Read the model definition and answer for the solid it produces. Units are mm, in the model's axes. A direction names the side the tool comes from. Give positions to 0.01 mm unless a question says otherwise; leave off trailing zeros. Loops run counter-clockwise (first coordinate to the right, second up) from the corner with the lowest first, then second, coordinate; pieces in that order, holes last. Notation, with made-up numbers: (7.25, -35.5) - (57.25, -35.5) arc R31 ccw to (57.25, -5.5) - close; hole circle Ø11 at (57.5, 6.25). An arc over 180 degrees is marked (long way). Put each result on its own line as item: value. Start each with the question number.
1. For faces 4 (the cylindrical face through (78.4, 0.18, 46.79)), 5 (the flat face through (76.835, -26, -25)), determine the directions among +Z, -Z, +X, -X, +Y, -Y from which every point of the face is accessible in a straight line to the end or side of a thin tool.
2. For a pull along Z with two mould halves and no side action, classify faces 1 (the flat face through (67.31, -18, 65)), 2 (the flat face through (80.01, 44, 1)), 3 (the cylindrical face through (1.12, -22.025, -99.184)) as released by +Z, released by -Z, zero draft, split by the parting line, or undercut.
3. Given pin 1 Ø6 at (x, z) = (13.5, 31) entering from -Y; pin 2 Ø8 at (x, y) = (-53, 69) entering from -Z; pin 3 Ø2 at (x, z) = (36.5, 64) entering from +Y; pin 4 Ø7 at (y, z) = (0, -50.8) entering from -X, each flat-ended and moving along its own axis, determine where each tip first touches the part or whether it passes through.
4. A cutting plane is placed at A-A, the plane y = 0. Determine the outline of the cut face in (x, z) (3 decimals), plus the area to 3 significant figures.
5. Consider L1, parallel to X at y = -4.5, z = 46.5 (3 decimals); L2, parallel to Y at x = 49.5, z = 4.5; L3, parallel to X at y = 68, z = -7. Determine where each line is inside the solid, lowest interval first. Write a range as from..to.
6. A cutting plane is placed at C-C, the plane x = -46.5. Determine the outline of the cut face in (y, z) (3 decimals), plus the area to 3 significant figures.
Autodesk Inventor part; units mm, degrees
ref_plane "YZ Plane" through (0, 0, 0) normal (1, 0, 0) x (0, 1, 0)
ref_plane "XZ Plane" through (0, 0, 0) normal (0, 1, 0) x (-1, 0, 0)
ref_plane "XY Plane" through (0, 0, 0) normal (0, 0, 1) x (1, 0, 0)
sketch "Sketch1" plane through (0, 0, 0) normal (0, 0, 1) x (1, 0, 0)
  line L0 (-179.5854, 0) -> (123.2759, 0)
  line L1 (0, -20.32) -> (0, 121.92)
  line L2 (-80.01, 101.6) -> (80.01, 101.6)
  line L3 (80.01, 50.8) -> (-80.01, 50.8) construction
  line L4 (80.01, 0) -> (-136.3195, 0) construction
  arc A0 (-80.01, 101.6) -> (-76.835, 98.425) centre (-76.835, 101.6) ccw
  line L5 (60.96, 85.725) -> (-64.135, 85.725)
  arc A1 (-76.835, 98.425) -> (-64.135, 85.725) centre (-64.135, 98.425) ccw
  arc A2 (67.31, 66.675) -> (76.835, 57.15) centre (76.835, 66.675) ccw
  arc A3 (67.31, 79.375) -> (60.96, 85.725) centre (60.96, 79.375) ccw
  line L6 (67.31, 79.375) -> (67.31, 66.675)
  line L7 (80.01, 101.6) -> (80.01, 0)
  line L8 (80.01, 98.425) -> (-76.835, 98.425) construction
  line L9 (-64.135, 85.725) -> (-64.135, 101.6) construction
  line L10 (-76.835, 98.425) -> (-76.835, 101.6) construction
  line L11 (60.96, 85.725) -> (80.01, 85.725) construction
  line L12 (67.31, 79.375) -> (80.01, 79.375) construction
  line L13 (60.96, 50.8) -> (60.96, 101.6) construction
  line L14 (67.31, 66.675) -> (80.01, 66.675) construction
  line L15 (76.835, 57.15) -> (76.835, 0)
  line L16 (76.835, 57.15) -> (80.01, 57.15) construction
  line L17 (76.835, 0) -> (80.01, 0)
  point P0 (0, 0)
  point P1 (0, 101.6)
  dimension "d0" = 101.6
  dimension "d2" = 160.02
  dimension "d4" = 50.8
  dimension "d10" = 6.35
  dimension "d11" = 12.7
  dimension "d13" = 3.175
  dimension "d14" = 34.925
  dimension "d15" = 19.05
  dimension "d16" = 12.7
revolve "Revolution1" add sketch "Sketch1" angle 360 about axis through (-10, 0, 0) along (1, 0, 0) contours L15 A2 L6 A3 L5 L1 L2 L7 L0 | L5 A1 A0 L2 L1
sketch "Sketch2" plane through (76.835, 0, 0) normal (-1, 0, 0) x (0, 0, 1)
  circle A0 centre (0, 0) radius 57.15
  circle A1 centre (0, 0) radius 50.8 construction
  circle A2 centre (0, 0) radius 34.925
  circle A3 centre (0, 50.8) radius 4.0132
  circle A4 centre (-50.8, 0) radius 4.0132
  circle A5 centre (0, -50.8) radius 4.0132
  circle A6 centre (50.8, 0) radius 4.0132
  dimension "d18" = 101.6
  dimension "d19" = 69.85
  dimension "d20" = 8.0264
  dimension "d23" = 360
extrude "Extrusion1" cut sketch "Sketch2" against normal through all contours A2 | A3 | A4 | A5 | A6
properties part number "rim_8 in x 6.3 in"
Return value:
1. face 4: +X, -X
1. face 5: -X
2. face 1: undercut
2. face 2: zero draft
2. face 3: split by the parting line
3. pin 1: stops at y = -97.67
3. pin 2: stops at z = -78.09
3. pin 3: stops at y = 79.71
3. pin 4: passes through
4. outline: (-80.01, -101.6) - (80.01, -101.6) - (80.01, -54.813) - (76.835, -54.813) - (76.835, -57.15) arc R9.525 ccw to (67.31, -66.675) - (67.31, -79.375) arc R6.35 cw to (60.96, -85.725) - (-64.135, -85.725) arc R12.7 ccw to (-76.835, -98.425) arc R3.175 ccw to start; (-80.01, 101.6) arc R3.175 ccw to (-76.835, 98.425) arc R12.7 ccw to (-64.135, 85.725) - (60.96, 85.725) arc R6.35 cw to (67.31, 79.375) - (67.31, 66.675) arc R9.525 ccw to (76.835, 57.15) - (76.835, 54.813) - (80.01, 54.813) - (80.01, 101.6) - close; (76.835, -46.787) - (80.01, -46.787) - (80.01, -34.925) - (76.835, -34.925) - close; (76.835, 34.925) - (80.01, 34.925) - (80.01, 46.787) - (76.835, 46.787) - close
4. area: 5,720 mm2
5. L1: x = 76.835..80.01
5. L2: y = -101.5..-85.61, 85.61..101.5
5. L3: x = 67.31..80.01
6. outline: circle Ø203.2 at (0, 0); hole circle Ø171.45 at (0, 0)
6. area: 9,340 mm2
